Check sheet for the modelled part. Datum: model origin and axes. Units: mm. A direction names the side the tool comes from. Round coordinates to 2 decimals unless told otherwise and drop trailing zeros. Write each loop counter-clockwise with the first axis right and the second up, starting at its lowest first coordinate (ties: lowest second). Pieces come first, ordered by that corner, then holes. Notation, with made-up numbers: (22.25, 38.5) - (71.25, 38.5) arc R10 cw to (71.25, 51.5) - close; hole circle Ø9 at (18, 20.25). An arc over 180 degrees is marked (long way). Answer as a JSON object with one key per item and string values. Group by question number.
Item 1: Thickness scan on line 1 (Y direction, x = -1.6, z = -0.6); line 2 (Z direction, x = -0.45, y = 1.25); line 3 (X direction, y = 1.25, z = 1.05). Record the ranges inside material, lowest first.
Item 2: Set-up check for faces 1 (the cylindrical face through (-1.5, -2.34, 0.07)), 2 (the flat face through (-0.842, 1.527, 0.373)), 3 (the flat face through (0, -5, 0)): record each of +Z, -Z, +X, -X, +Y, -Y from which the full face is reachable in a straight line by a thin tool's end or side.
Item 3: Sectioned sample at B-B on z = 0. Record the boundary of the cut face in (x, y), plus the area to 3 significant figures.
Item 4: Sectioned sample at A-A on x = 0. Record the boundary of the cut face in (y, z), plus the area to 3 significant figures.
Item 5: Release check for a two-part mould opening along Z. For faces 4 (the flat face through (0, 1, 0)), 5 (the flat face through (1, 2, 1)), 6 (the cylindrical face through (-0.54, 0.87, 2.44)) record: pulls with the +Z half, pulls with the -Z half, needs draft (parallel to the pull), parting line crosses it, or undercut.
Item 6: Sectioned sample at C-C on y = -2.75. Record the boundary of the cut face in (x, z).
Item 7: Gauge pin test, flat ends, axial feed: P1, Ø1.5, axis at x = -0.5, z = -2, coming from the -Y side; P2, Ø1.4, axis at x = 0, z = -0.5, coming from the +Y side; P3, Ø1.5, axis at x = -1.5, y = 0, coming from the -Z side. Record the tip position at first contact, or that the pin passes through.
```python
from build123d import *

# Parameters (mm, degrees)
CROQUIS1_R              = 2.5
SALIENTE_EXTRUIR1_DEPTH = 2
CROQUIS2_R              = 1.5
SALIENTE_EXTRUIR2_DEPTH = 5
CHAFL_N1_SIZE           = 0.25
REDONDEO1_R             = 0.5
CORTAR_EXTRUIR1_DEPTH   = 1
CHAFL_N2_SIZE           = 0.25
CHAFL_N2_SIZE2          = 0.933012702


with BuildPart() as part:
    # Croquis1 → Saliente-Extruir1 (new body)
    with BuildSketch(Plane(origin=(0, 0, 0), x_dir=(1, 0, 0), z_dir=(0, 1, 0))):
        Circle(CROQUIS1_R)
    extrude(amount=SALIENTE_EXTRUIR1_DEPTH)

    # Croquis2 → Saliente-Extruir2 (add)
    with BuildSketch(Plane.XZ):
        Circle(CROQUIS2_R)
    extrude(amount=SALIENTE_EXTRUIR2_DEPTH)

    # Chaflán1
    chafl_n1_edges = [part.edges().sort_by_distance(p)[0] for p in [
        (-2.5, 0, 0),
        (-1.5, -5, 0),
    ]]
    chamfer(chafl_n1_edges, length=CHAFL_N1_SIZE)

    # Redondeo1
    redondeo1_edges = [part.edges().sort_by_distance(p)[0] for p in [
        (-2.5, 2, 0),
    ]]
    fillet(redondeo1_edges, radius=REDONDEO1_R)

    # Croquis3 → Cortar-Extruir1 (cut)
    with BuildSketch(Plane(origin=(0, 2, 0), x_dir=(1, 0, 0), z_dir=(0, 1, 0))):
        Polygon((0.25, 0.25), (1.45, 0.25), (1.45, -0.25), (0.25, -0.25), (0.25, -1.45), (-0.25, -1.45), (-0.25, -0.25), (-1.45, -0.25), (-1.45, 0.25), (-0.25, 0.25), (-0.25, 1.45), (0.25, 1.45), align=None)
    extrude(amount=-CORTAR_EXTRUIR1_DEPTH, mode=Mode.SUBTRACT)

    # Chaflán2
    chafl_n2_edges = [part.edges().sort_by_distance(p)[0] for p in [
        (-0.25, 2, -0.85),
        (-0.85, 2, -0.25),
        (-0.85, 2, 0.25),
        (-0.25, 2, 0.85),
        (0.25, 2, 0.85),
        (0.85, 2, 0.25),
        (0.85, 2, -0.25),
        (0.25, 2, -0.85),
    ]]
    chafl_n2_side = [part.faces().sort_by_distance(p)[0] for p in [
        (-1.943431458, 2, 0),
    ]]
    chamfer(chafl_n2_edges, length=CHAFL_N2_SIZE, length2=CHAFL_N2_SIZE2, reference=chafl_n2_side[0])


solid = part.part
```
Completed:
{
 "1": {"line 1": "0 to 2", "line 2": "-2.46 to -0.3, 0.3 to 2.46", "line 3": "-2.27 to -0.3, 0.3 to 2.27"},
 "2": {"face 1": "-Y", "face 2": "+Y", "face 3": "+Z, -Z, +X, -X, -Y"},
 "3": {"outline": "(-2.5, 0.25) - (-2.25, 0) - (-1.5, 0) - (-1.5, -4.75) - (-1.25, -5) - (1.25, -5) - (1.5, -4.75) - (1.5, 0) - (2.25, 0) - (2.5, 0.25) - (2.5, 1.5) arc R0.5 ccw to (2, 2) - (1.45, 2) - (1.45, 1) - (-1.45, 1) - (-1.45, 2) - (-2, 2) arc R0.5 ccw to (-2.5, 1.5) - close", "area": "21.9 mm²"},
 "4": {"outline": "(-5, -1.25) - (-4.75, -1.5) - (0, -1.5) - (0, -2.25) - (0.25, -2.5) - (1.5, -2.5) arc R0.5 ccw to (2, -2) - (2, -1.45) - (1, -1.45) - (1, 1.45) - (2, 1.45) - (2, 2) arc R0.5 ccw to (1.5, 2.5) - (0.25, 2.5) - (0, 2.25) - (0, 1.5) - (-4.75, 1.5) - (-5, 1.25) - close", "area": "21.9 mm²"},
 "5": {"face 4": "undercut", "face 5": "needs draft", "face 6": "parting line crosses it"},
 "6": {"outline": "circle Ø3 at (0, 0)"},
 "7": {"P1": "y = -4.94", "P2": "y = 2", "P3": "z = -2.37"}
}
